Model file for the job. Use its own axes, mm. A direction names the side the tool comes from. Give positions to 0.01 mm unless a question says otherwise; leave off trailing zeros. Order: outer loops, then holes, each group sorted by start corner. A loop starts at its lowest first (then second) coordinate and runs counter-clockwise, first axis right, second up. Notation, with made-up numbers: (83.5, 81) -> (124.5, 81) arc R25 ccw to (124.5, 100) -> close; hole circle Ø6 at (27.25, 8). An arc over 180 degrees is marked (long way). Use CSV: the item, a comma, the result in double quotes. Start each with the question number.
1. Pull direction X, two halves, no side cores. Call faces 1 (the flat face through (-571.5, 25, -125)), 2 (the cylindrical face through (-397.12, 5.01, -231.09)), 3 (the flat face through (-282, 25, 0)): released by +X, released by -X, zero draft, split by the parting line, or undercut.
2. 3-axis set-ups, long thin cutter, end or side, ignore diameter. For faces 4 (the cylindrical face through (-299.587, 30.196, -177.862)), 5 (the cylindrical face through (-143.167, 5.009, -217.782)): which of +Z, -Z, +X, -X, +Y, -Y reach the whole face in a straight line?
3. Wall check: line 1 (X direction, y = 39, z = -180); line 2 (Z direction, x = -398, y = 35); line 3 (X direction, y = 2.75, z = -180.34). Give the ranges that are in metal, low to high. Write a range as from..to.
4. Cut at C-C on x = -102. List the corners of the cut face in (y, z).
5. Cut at A-A on z = -156.5. List the corners of the cut face in (x, y).
6. Cut at B-B on y = 17. Give the number of separate pieces and of enclosed holes in the cut face, then the cut area to 3 significant figures.
```python
from build123d import *

# Parameters (mm, degrees)
BOSS_EXTRUDE1_DEPTH = 50.8
SKETCH2_R           = 50.8
CUT_EXTRUDE1_DEPTH  = 10.16
SKETCH3_R           = 11.43
CUT_EXTRUDE2_DEPTH  = 627.721516784


with BuildPart() as part:
    # Sketch1 → Boss-Extrude1 (new body)
    with BuildSketch(Plane(origin=(0, 0, 0), x_dir=(1, 0, 0), z_dir=(0, 1, 0))):
        with BuildLine():
            Line((-12.7, 0), (-558.8, 0))
            ThreePointArc((-558.8, 0), (-567.780256121, 3.719743879), (-571.5, 12.7))
            Line((-571.5, 12.7), (-571.5, 241.3))
            ThreePointArc((-571.5, 241.3), (-567.780256121, 250.280256121), (-558.8, 254))
            Line((-558.8, 254), (-12.7, 254))
            ThreePointArc((-12.7, 254), (-3.719743879, 250.280256121), (0, 241.3))
            Line((0, 241.3), (0, 12.7))
            ThreePointArc((0, 12.7), (-3.719743879, 3.719743879), (-12.7, 0))
        make_face()
    extrude(amount=BOSS_EXTRUDE1_DEPTH)

    # Sketch2 → Cut-Extrude1 (cut)
    with BuildSketch(Plane(origin=(0, 0, 0), x_dir=(1, 0, 0), z_dir=(0, 1, 0))):
        with Locations(Location((-177.499611663, 66.04, 0), (0, 0, 270))):
            Circle(SKETCH2_R)
        with Locations(Location((-66.57081555, 66.04, 0), (0, 0, 270))):
            Circle(SKETCH2_R)
        with Locations(Location((-288.428407775, 66.04, 0), (0, 0, 270))):
            Circle(SKETCH2_R)
        with Locations(Location((-399.357203888, 66.04, 0), (0, 0, 270))):
            Circle(SKETCH2_R)
        with Locations(Location((-510.286, 66.04, 0), (0, 0, 270))):
            Circle(SKETCH2_R)
        with Locations(Location((-177.499611663, 180.34, 0), (0, 0, 270))):
            Circle(SKETCH2_R)
        with Locations(Location((-288.428407775, 180.34, 0), (0, 0, 270))):
            Circle(SKETCH2_R)
        with Locations(Location((-399.357203888, 180.34, 0), (0, 0, 270))):
            Circle(SKETCH2_R)
        with Locations(Location((-510.286, 180.34, 0), (0, 0, 270))):
            Circle(SKETCH2_R)
        with Locations(Location((-66.57081555, 180.34, 0), (0, 0, 270))):
            Circle(SKETCH2_R)
    extrude(amount=CUT_EXTRUDE1_DEPTH, mode=Mode.SUBTRACT)

    # Sketch3 → Cut-Extrude2 (cut, through all)
    with BuildSketch(Plane.XZ.offset(-10.16)):
        with Locations(Location((-66.57081555, -180.34, 0), (0, 0, 270))):
            Circle(SKETCH3_R)
        with Locations(Location((-177.499611663, -180.34, 0), (0, 0, 270))):
            Circle(SKETCH3_R)
        with Locations(Location((-288.428407775, -180.34, 0), (0, 0, 270))):
            Circle(SKETCH3_R)
        with Locations(Location((-399.357203888, -180.34, 0), (0, 0, 270))):
            Circle(SKETCH3_R)
        with Locations(Location((-510.286, -180.34, 0), (0, 0, 270))):
            Circle(SKETCH3_R)
        with Locations(Location((-510.286, -66.04, 0), (0, 0, 90))):
            Circle(SKETCH3_R)
        with Locations(Location((-399.357203888, -66.04, 0), (0, 0, 90))):
            Circle(SKETCH3_R)
        with Locations(Location((-288.428407775, -66.04, 0), (0, 0, 90))):
            Circle(SKETCH3_R)
        with Locations(Location((-177.499611663, -66.04, 0), (0, 0, 90))):
            Circle(SKETCH3_R)
        with Locations(Location((-66.57081555, -66.04, 0), (0, 0, 90))):
            Circle(SKETCH3_R)
    extrude(amount=-CUT_EXTRUDE2_DEPTH, mode=Mode.SUBTRACT)


solid = part.part
```
Verdict:
1,face 1,"released by -X"
1,face 2,"undercut"
1,face 3,"zero draft"
2,face 4,"+Y, -Y"
2,face 5,"-Y"
3,line 1,"-571.5..-521.71, -498.86..-410.78, -387.93..-299.85, -277..-188.92, -166.07..-78, -55.15..0"
3,line 2,"-254..-191.69, -168.99..-77.39, -54.69..0"
3,line 3,"-571.5..-561.09, -459.49..-450.16, -348.56..-339.23, -237.63..-228.3, -126.7..-117.37, -15.77..0"
4,outline,"(0, -254) -> (50.8, -254) -> (50.8, 0) -> (0, 0) -> (0, -29.63) -> (10.16, -29.63) -> (10.16, -102.45) -> (0, -102.45) -> (0, -143.93) -> (10.16, -143.93) -> (10.16, -216.75) -> (0, -216.75) -> close"
5,outline,"(-571.5, 0) -> (-555.14, 0) -> (-555.14, 10.16) -> (-465.43, 10.16) -> (-465.43, 0) -> (-444.22, 0) -> (-444.22, 10.16) -> (-354.5, 10.16) -> (-354.5, 0) -> (-333.29, 0) -> (-333.29, 10.16) -> (-243.57, 10.16) -> (-243.57, 0) -> (-222.36, 0) -> (-222.36, 10.16) -> (-132.64, 10.16) -> (-132.64, 0) -> (-111.43, 0) -> (-111.43, 10.16) -> (-21.71, 10.16) -> (-21.71, 0) -> (0, 0) -> (0, 50.8) -> (-571.5, 50.8) -> close"
6,separate pieces,"1"
6,enclosed holes,"10"
6,area,"141,000 mm^2"
